The listing builds one solid part. Answer for the finished solid, in the listing's coordinates (mm). Face numbers are marked on the shaded views. A direction names the side the tool comes from. Coordinates: 2 decimals unless noted, no trailing zeros. Loops run counter-clockwise (first coordinate to the right, second up) from the corner with the lowest first, then second, coordinate; pieces in that order, holes last. Notation, with made-up numbers: M 60.25,42 L 91.25,42 A16 ccw 91.25,49 Z; hole C 86.5,47.5 d5. An arc over 180 degrees is marked long. Return JSON: item names as keys, results as strings. Group by question number.
1. Section A-A (z = -63) is taken. Write down the section's boundary in (x, y).
2. Which of the six approach directions +Z, -Z, +X, -X, +Y, -Y give full straight-line access (tool end or side, diameter ignored) to the marked faces 1 and 2?
3. Straight lines are drawn through the part: L1, parallel to Y at x = 0, z = -22.75; L2, parallel to Y at x = 16, z = -7.5; L3, parallel to Z at x = 76, y = 41. For each, find the intervals that lie inside material, in ascending order. Write a range as from..to.
4. Given P1, Ø8, axis at x = 28.5, y = 7, coming from the +Z side; P2, Ø2.5, axis at x = -59, y = 58, coming from the +Z side; P3, Ø1.5, axis at y = 12.5, z = -18.5, coming from the -X side; P4, Ø10, axis at x = 26.5, y = 3, coming from the -Z side, each flat-ended and moving along its own axis, determine where each tip first touches the part or whether it passes through.
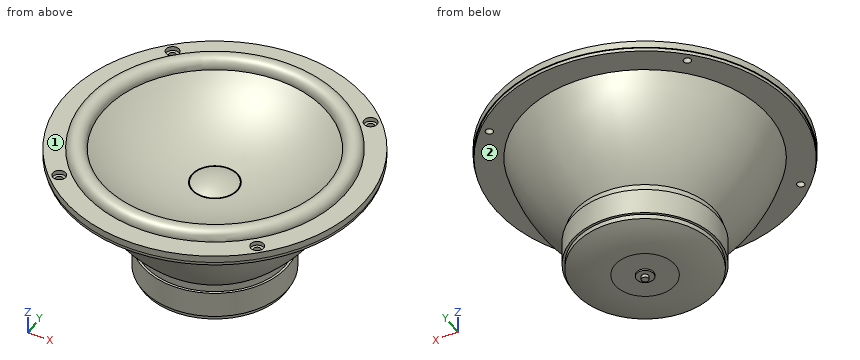
```python
from build123d import *

# Parameters (mm, degrees)
SKETCH3_R          = 2.15
CUT_HOLES_DEPTH    = 152.160973799
SKETCH4_R          = 3.7973
CUT_EXTRUDE4_DEPTH = 2.5019


with BuildPart() as part:
    # Sketch1 → Revolve1 (revolve)
    with BuildSketch(Plane(origin=(0, 0, 0), x_dir=(1, 0, 0), z_dir=(0, 1, 0))):
        with BuildLine():
            Line((76.360050956, 0), (88, 0))
            Line((88, 0), (88, 4.1))
            Line((88, 4.1), (87.5, 4.1))
            Line((87.5, 4.1), (87.5, 6.1))
            Line((87.5, 6.1), (72.25, 6.1))
            ThreePointArc((72.25, 6.1), (60.431927794, 33.612739382), (41.107075762, 56.4856))
            Line((41.107075762, 56.4856), (41.107075762, 60.8036))
            Line((41.107075762, 60.8036), (42.5, 60.8036))
            Line((42.5, 60.8036), (42.5, 75.942))
            Line((42.5, 75.942), (41.107075762, 75.942))
            Line((41.107075762, 75.942), (41.107075762, 78.736))
            ThreePointArc((41.107075762, 78.736), (29.490355709, 81.776565788), (17.526, 82.8))
            Line((17.526, 82.8), (5, 82.8))
            Line((5, 82.8), (5, 83.8))
            Line((5, 83.8), (2, 83.8))
            Line((2, 83.8), (2, 85.8))
            Line((2, 85.8), (0, 85.8))
            Line((0, 85.8), (0, 19.240383034))
            ThreePointArc((0, 19.240383034), (6.644837955, 19.937889067), (13, 22))
            Line((13, 22), (13, 23))
            Line((13, 23), (13.5, 23))
            Line((13.5, 23), (13.5, 22))
            ThreePointArc((13.5, 22), (40.947327355, 15.0380389), (65.342731977, 0.661359359))
            ThreePointArc((65.342731977, 0.661359359), (70.501977385, -5.490068668), (76.360050956, 0))
        make_face()
    revolve(axis=Axis((0, 0, -19.240383034), (0, 0, -1)))

    # Sketch3 → Cut holes (cut, through all)
    with BuildSketch(Plane.XY):
        with Locations((-58.336309448, 58.336309448)):
            Circle(SKETCH3_R)
        with Locations((58.336309448, 58.336309448)):
            Circle(SKETCH3_R)
        with Locations((58.336309448, -58.336309448)):
            Circle(SKETCH3_R)
        with Locations((-58.336309448, -58.336309448)):
            Circle(SKETCH3_R)
    extrude(amount=-CUT_HOLES_DEPTH, mode=Mode.SUBTRACT)

    # Sketch4 → Cut-Extrude4 (cut)
    with BuildSketch(Plane.XY):
        with Locations((-58.336309448, 58.336309448)):
            Circle(SKETCH4_R)
        with Locations((58.336309448, 58.336309448)):
            Circle(SKETCH4_R)
        with Locations((58.336309448, -58.336309448)):
            Circle(SKETCH4_R)
        with Locations((-58.336309448, -58.336309448)):
            Circle(SKETCH4_R)
    extrude(amount=-CUT_EXTRUDE4_DEPTH, mode=Mode.SUBTRACT)


solid = part.part
```
Worked out:
{
 "1": {"outline": "C 0,0 d85"},
 "2": {"face 1": "+Z", "face 2": "-Z"},
 "3": {"L1": "-66.27..-13.5, -13..13, 13.5..66.27", "L2": "-70.07..-53.32, 53.32..70.07", "L3": "-6.1..0"},
 "4": {"P1": "z = -17.81", "P2": "through", "P3": "x = -67.29", "P4": "z = -82.68"}
}
